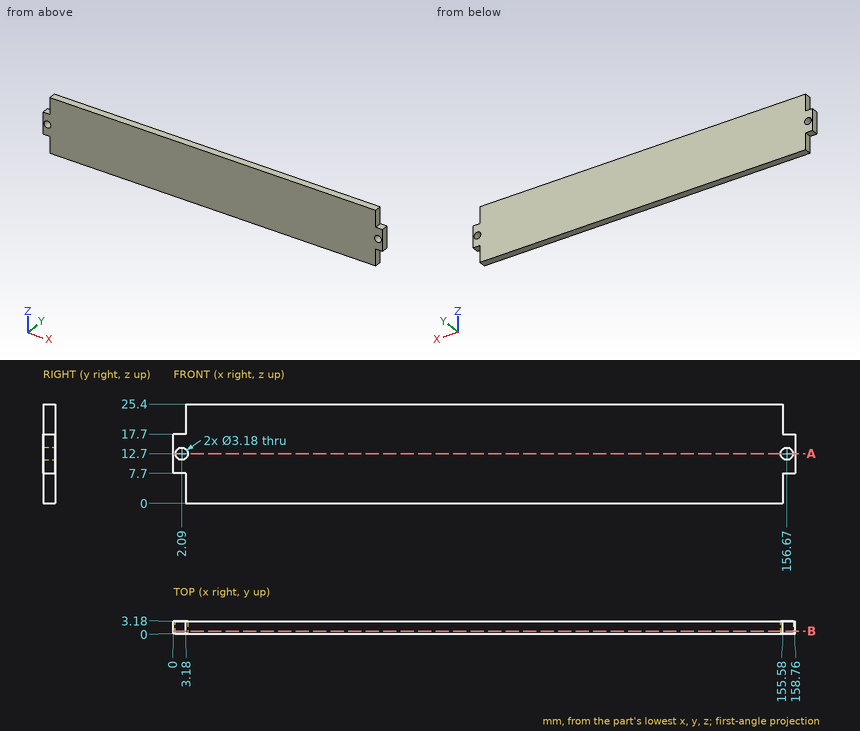
Could you check a few things on this drawing? It's one solid part, dimensions in mm from its lowest x, y, z. Coordinates: 2 decimals unless noted, no trailing zeros. Loops run counter-clockwise (first coordinate to the right, second up) from the corner with the lowest first, then second, coordinate; pieces in that order, holes last. Notation, with made-up numbers: (75, -31.5) - (117, -31.5) arc R21 ccw to (117, -8.5) - close; hole circle Ø6 at (69, 57). An arc over 180 degrees is marked (long way). Answer as a JSON object with one key per item and string values. Group by question number.
Item 1: If we section it at A-A (z = 12.7): List the corners of the cut face in (x, y) for me.
Item 2: If we section it at B-B (y = 0.7): List the corners of the cut face in (x, z) for me.
Item 3: If I drill on L1, parallel to X at y = 1.6, z = 12.7; L2, parallel to Z at x = 2.09, y = 0.75; L3, parallel to X at y = 1.25, z = 23.75, over which ranges is the centre line in solid material (lowest first)? Write a range as from..to.
Item 4: For pin 1 (1.6 mm diameter, centred on x = 157.5, y = 2, fed in from +Z); pin 2 (1.6 mm diameter, centred on y = 2, z = 23, fed in from +X); pin 3 (1.9 mm diameter, centred on x = 156.67, z = 12.7, fed in from -Y), each with a flat end and sliding along its axis, tell me the tip position at first contact or that it passes through.
Returned:
{
 "1": {"outline": "(0, 0) - (0.5, 0) - (0.5, 3.18) - (0, 3.18) - close; (3.68, 0) - (155.08, 0) - (155.08, 3.18) - (3.68, 3.18) - close; (158.26, 0) - (158.76, 0) - (158.76, 3.18) - (158.26, 3.18) - close"},
 "2": {"outline": "(0, 7.7) - (3.18, 7.7) - (3.18, 0) - (155.58, 0) - (155.58, 7.7) - (158.76, 7.7) - (158.76, 17.7) - (155.58, 17.7) - (155.58, 25.4) - (3.18, 25.4) - (3.18, 17.7) - (0, 17.7) - close; hole circle Ø3.18 at (2.09, 12.7); hole circle Ø3.18 at (156.67, 12.7)"},
 "3": {"L1": "x = 0..0.5, 3.68..155.08, 158.26..158.76", "L2": "z = 7.7..11.11, 14.29..17.7", "L3": "x = 3.18..155.58"},
 "4": {"pin 1": "stops at z = 17.7", "pin 2": "stops at x = 155.58", "pin 3": "passes through"}
}
